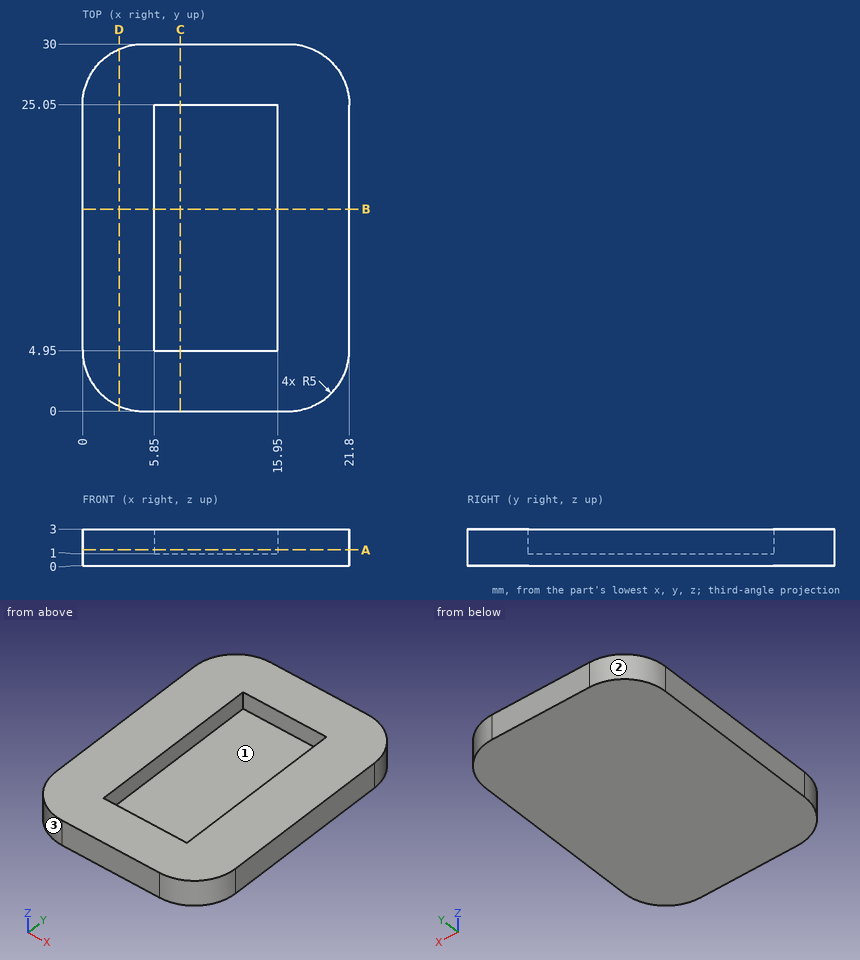
Input: dimensioned drawing with shaded views. Units: mm. Origin: part minimum x, y, z. Coordinates: 2 decimals unless noted, no trailing zeros. Loops run counter-clockwise (first coordinate to the right, second up) from the corner with the lowest first, then second, coordinate; pieces in that order, holes last.
Q1. Line query: line 1 along X through (y, z) = (6, 1.7); line 2 along Y through (x, z) = (15, 2.95); line 3 along Z through (x, y) = (15, 18.25). Output: solid intervals per line, ascending.
Results are:
line 1: x = 0 to 5.85, 15.95 to 21.8
line 2: y = 0 to 4.95, 25.05 to 30
line 3: z = 0 to 1
Q2. Section B-B, the plane y = 16.5. Return the cut outline in (x, z).
Results are:
outline: (0, 0) - (21.8, 0) - (21.8, 3) - (15.95, 3) - (15.95, 1) - (5.85, 1) - (5.85, 3) - (0, 3) - close
Q3. Section A-A, the plane z = 1.3. Return the cut outline in (x, y).
Results are:
outline: (0, 5) arc R5 ccw to (5, 0) - (16.8, 0) arc R5 ccw to (21.8, 5) - (21.8, 25) arc R5 ccw to (16.8, 30) - (5, 30) arc R5 ccw to (0, 25) - close; hole (5.85, 4.95) - (15.95, 4.95) - (15.95, 25.05) - (5.85, 25.05) - close
Q4. Section D-D, the plane x = 3. Return the cut outline in (y, z), and give its area (3 significant figures).
Results are:
outline: (0.42, 0) - (29.58, 0) - (29.58, 3) - (0.42, 3) - close
area: 87.5 mm2
Q5. Contact query for flat-ended pins moving along their axis: pin 1 (3 mm diameter, centred on x = 9, y = 11.5, fed in from +Z); pin 2 (1.5 mm diameter, centred on x = 18.5, z = 2.5, fed in from -Y). Output: stop coordinate, or through.
Results are:
pin 1: stops at z = 1
pin 2: stops at y = 0.09
Q6. Mould query, pull axis Y, two halves, no side actions, for the marked faces 1, 2 and 3. Classes: +Y half, -Y half, draft (parallel to the pull), parting line (faces both ways), or undercut.
Results are:
face 1: undercut
face 2: +Y half
face 3: -Y half
Q7. Section C-C, the plane x = 8. Return the cut outline in (y, z).
Results are:
outline: (0, 0) - (30, 0) - (30, 3) - (25.05, 3) - (25.05, 1) - (4.95, 1) - (4.95, 3) - (0, 3) - close
